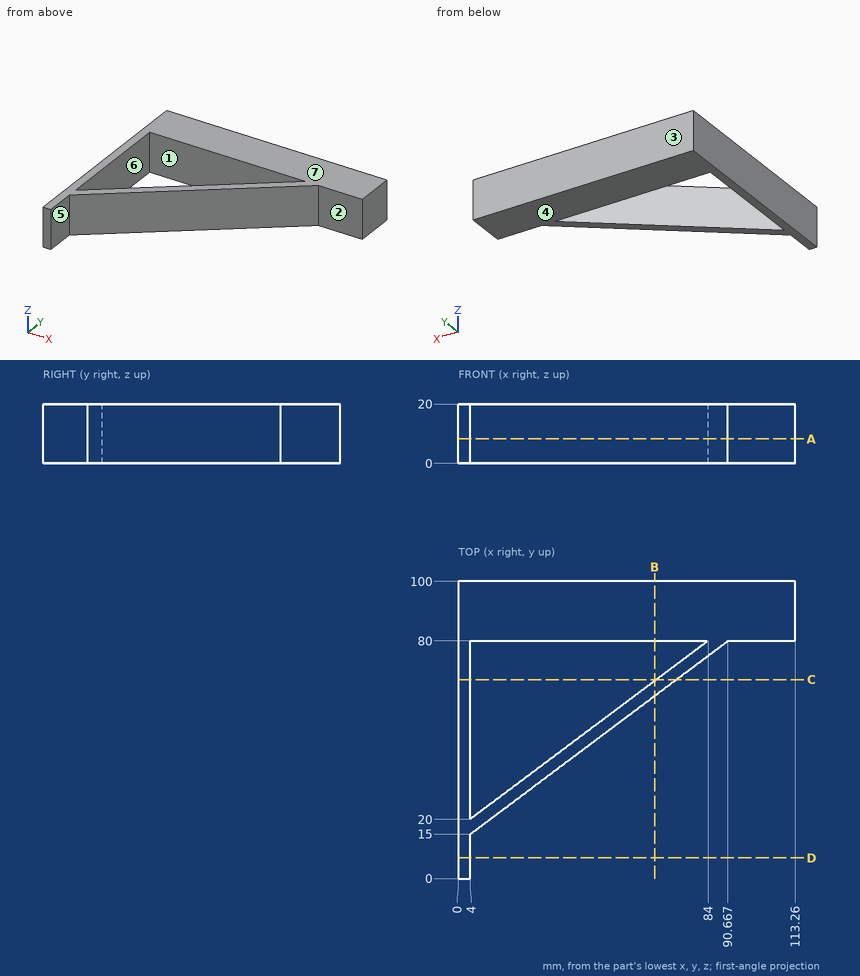
Source: three-view drawing plus pictorial views. Frame: mm from the lowest corner of the part. A direction names the side the tool comes from. Round coordinates to 2 decimals unless told otherwise and drop trailing zeros. Order: outer loops, then holes, each group sorted by start corner. A loop starts at its lowest first (then second) coordinate and runs counter-clockwise, first axis right, second up. Notation, with made-up numbers: (-34, 1.25) -> (-5, 1.25) arc R32 cw to (-5, 37.25) -> close; hole circle Ø6 at (-4.75, -17.5). An arc over 180 degrees is marked (long way). Use CSV: the item, a comma, the result in double quotes. Start each with the question number.
1) Section D-D (y = 7). Return the cut outline in (x, z).
2) Draft query along Y for the marked faces 1, 2, 3 and 4. Return one class per face: +Y half, -Y half, draft (parallel to the pull), parting line (faces both ways), or undercut.
3) Set-up query: the marked faces 5, 6 and 7. Return all of +Z, -Z, +X, -X, +Y, -Y with unobstructed straight access to the full face (end or side cutting, diameter ignored); none if empty.
4) Section B-B (x = 66). Return the cut outline in (y, z).
5) Section C-C (y = 67). Return the cut outline in (x, z), and give its area (3 significant figures).
6) Section A-A (z = 8.25). Return the cut outline in (x, y).
7) Material intervals for line 1 along X through (y, z) = (70, 1) (1 decimal); line 2 along X through (y, z) = (28.5, 18.5) (1 decimal); line 3 along Y through (x, z) = (10.5, 2) (1 decimal), sorted ascending. Write a range as from..to.
8) First-contact query: pin 1 Ø6 at (y, z) = (57.5, 6.5) entering from +X (1 decimal); pin 2 Ø4 at (y, z) = (76.5, 4.5) entering from +X (1 decimal); pin 3 Ø10 at (x, z) = (42.5, 6) entering from -Y (1 decimal). Flat tips, straight axial feed; report the tip coordinate or a pass-through.
Returned:
1,outline,"(0, 0) -> (4, 0) -> (4, 20) -> (0, 20) -> close"
2,face 1,"undercut"
2,face 2,"-Y half"
2,face 3,"+Y half"
2,face 4,"draft"
3,face 5,"+Z, -Z, +X, -Y"
3,face 6,"+Z, -Z"
3,face 7,"+Z, +X, -X, +Y, -Y"
4,outline,"(61.5, 0) -> (66.5, 0) -> (66.5, 20) -> (61.5, 20) -> close; (80, 0) -> (100, 0) -> (100, 20) -> (80, 20) -> close"
5,outline,"(0, 0) -> (4, 0) -> (4, 20) -> (0, 20) -> close; (66.67, 0) -> (73.33, 0) -> (73.33, 20) -> (66.67, 20) -> close"
5,area,"213 mm²"
6,outline,"(0, 0) -> (4, 0) -> (4, 15) -> (90.67, 80) -> (113.26, 80) -> (113.26, 100) -> (0, 100) -> close; hole (4, 20) -> (84, 80) -> (4, 80) -> close"
7,line 1,"x = 0..4, 70.7..77.3"
7,line 2,"x = 0..4, 15.3..22"
7,line 3,"y = 19.9..24.9, 80..100"
8,pin 1,"stops at x = 64.7"
8,pin 2,"stops at x = 88.7"
8,pin 3,"stops at y = 40.1"
